Autodesk Inventor part; units mm, degrees
ref_plane "YZ Plane" through (0, 0, 0) normal (1, 0, 0) x (0, 1, 0)
ref_plane "XZ Plane" through (0, 0, 0) normal (0, 1, 0) x (-1, 0, 0)
ref_plane "XY Plane" through (0, 0, 0) normal (0, 0, 1) x (1, 0, 0)
sketch "Sketch2" plane through (0, 0, 0) normal (0, 0, 1) x (1, 0, 0)
  line L0 (0, 0) -> (48.55, 0)
  line L1 (48.55, 0) -> (48.55, -13)
  line L2 (48.55, -13) -> (44.55, -13)
  line L3 (44.55, -13) -> (44.55, -4)
  line L4 (44.55, -4) -> (38.55, -4)
  line L5 (38.55, -4) -> (38.55, -7)
  line L6 (38.55, -7) -> (0, -7)
  line L7 (0, -7) -> (0, 0)
  dimension "d0" = 48.55
  dimension "d1" = 4
  dimension "d2" = 6
  dimension "d3" = 13
  dimension "d4" = 4
  dimension "d5" = 7
revolve "Revolution1" add sketch "Sketch2" angle 360 about axis through (0, -7, 0) along (0, 1, 0)
fillet "Fillet1" radius 3 1 edges at (-48.55, 0, 0)
sketch "Sketch3" plane through (0, -7, 0) normal (0, -1, 0) x (1, 0, 0)
  circle A0 centre (0, -19.55) radius 17
  circle A1 centre (0, 0) radius 38.55
  circle A2 centre (0, 19.55) radius 17
  dimension "d8" = 34
  dimension "d11" = 360
  dimension "d15" = 19.55
extrude "Extrusion1" cut sketch "Sketch3" against normal blind 5 contours A0 | A2
sketch "Sketch5" plane through (0, -7, 0) normal (0, -1, 0) x (1, 0, 0)
  circle A0 centre (20, 0) radius 6.25
  point P0 (0, 0)
  dimension "d16" = 12.5
  dimension "d17" = 20
extrude "Extrusion2" cut sketch "Sketch5" against normal through all
properties part number "lid-proto-v1"
Verification items for the finished model (mm, model axes). A direction names the side the tool comes from. Round coordinates to 2 decimals unless told otherwise and drop trailing zeros. Write each loop counter-clockwise with the first axis right and the second up, starting at its lowest first coordinate (ties: lowest second). Pieces come first, ordered by that corner, then holes. Notation, with made-up numbers: (19, 83) - (70, 83) arc R30 cw to (70, 114) - close; hole circle Ø2 at (52, -35.75). An arc over 180 degrees is marked (long way). Answer as a JSON object with one key per item and string values. Group by question number.
Q1. Thickness scan on line 1 (Z direction, x = 0, y = -5.35); line 2 (X direction, y = -7.75, z = 0); line 3 (Y direction, x = -12, z = -21.5). Record the ranges inside material, lowest first.
Q2. Section check B-B, the plane x = 0. Enter the section's corners in (y, z), plus the area to 3 significant figures.
Q3. Section check A-A, the plane y = -5.25. Enter the section's corners in (x, z), plus the area to 3 significant figures.
Q4. Mould release check, pull along X, two halves, no side actions. Record for faces 3 (the flat face through (-20, -4, -33.2)), 4 (the cylindrical face through (44.85, -8.07, -18.59)), 5 (the flat face through (-1, 0, -1)): released by +X, released by -X, zero draft, split by the parting line, or undercut.
Q5. Tool access check on faces 1 (the cylindrical face through (13.756, -3.549, 0.275)), 2 (the flat face through (0, -2, -19)). Record the directions out of +Z, -Z, +X, -X, +Y, -Y that give a thin tool (end or side, any length) a straight path to the whole face; none if there is none.
Q6. Go/stop test with flat-tipped pins: pin 1 Ø1.5 at (x, z) = (7, 28) entering from -Y; pin 2 Ø6 at (y, z) = (-5, -10) entering from +X; pin 3 Ø20 at (x, z) = (20, 0) entering from -Y. Record where each tip stops, or that it passes through.
Found:
{
 "1": {"line 1": "z = -48.55 to -44.55, -38.55 to -36.55, -2.55 to 2.55, 36.55 to 38.55, 44.55 to 48.55", "line 2": "x = -48.55 to -44.55, 44.55 to 48.55", "line 3": "y = -2 to 0"},
 "2": {"outline": "(-13, -48.55) - (-3, -48.55) arc R3 ccw to (0, -45.55) - (0, 45.55) arc R3 ccw to (-3, 48.55) - (-13, 48.55) - (-13, 44.55) - (-4, 44.55) - (-4, 38.55) - (-7, 38.55) - (-7, 36.55) - (-2, 36.55) - (-2, 2.55) - (-7, 2.55) - (-7, -2.55) - (-2, -2.55) - (-2, -36.55) - (-7, -36.55) - (-7, -38.55) - (-4, -38.55) - (-4, -44.55) - (-13, -44.55) - close", "area": "348 mm^2"},
 "3": {"outline": "circle Ø97.1 at (0, 0); circle Ø77.1 at (0, 0); hole circle Ø89.1 at (0, 0); hole circle Ø34 at (0, -19.55); hole circle Ø34 at (0, 19.55); hole circle Ø12.5 at (20, 0)", "area": "3,900 mm^2"},
 "4": {"face 3": "undercut", "face 4": "split by the parting line", "face 5": "zero draft"},
 "5": {"face 1": "+Y, -Y", "face 2": "-Y"},
 "6": {"pin 1": "stops at y = -2", "pin 2": "stops at x = 48.04", "pin 3": "stops at y = -7"}
}
